```python
from build123d import *

# Parameters (mm, degrees)
BOSS_EXTRUDE2_DEPTH            = 30
BOSS_EXTRUDE2_DEPTH_BACK       = 30
EXTRUDE_THIN2_START            = -25
EXTRUDE_THIN2_DEPTH            = 50
SKETCH2_W                      = 60
SKETCH2_H                      = 5
BOSS_EXTRUDE3_DEPTH            = 100
BOSS_EXTRUDE4_DEPTH            = 30
BOSS_EXTRUDE4_DEPTH_BACK       = 30
CUT_EXTRUDE2_REACH             = 143.361
SKETCH4_W                      = 60
SKETCH4_H                      = 5
CUT_EXTRUDE2_DIRECTION_2_REACH = 143.361
BOSS_EXTRUDE5_DEPTH            = 30
BOSS_EXTRUDE5_DEPTH_BACK       = 30
DRONE_ARM_FIT_CUT_DEPTH        = 50
CUT_EXTRUDE3_START             = -60
SKETCH8_W                      = 5
SKETCH8_H                      = 5
CUT_EXTRUDE3_DEPTH             = 60
SKETCH10_R                     = 13.15
CUT_EXTRUDE5_DEPTH             = 60


# Read off the part's stored shape, not the designer's step: Extrude-Thin2
with BuildPart() as part:
    # Sketch1 → Boss-Extrude2 (new, two sides: drawn at the far end of the back side and taken through both)
    with BuildSketch(Plane.XY.offset(-BOSS_EXTRUDE2_DEPTH_BACK)):
        Polygon((-13.01396445, -23.830717844), (13.01396445, -23.830717844), (55, -0.089432632), (55, 13.432214294), (-55, 13.432214294), (-55, -0.089432632), align=None)
    extrude(amount=BOSS_EXTRUDE2_DEPTH + BOSS_EXTRUDE2_DEPTH_BACK)

    # Extrude-Thin2 outline → Extrude-Thin2 (add)
    with BuildSketch(Plane.XY.offset(EXTRUDE_THIN2_START)):
        Polygon((50, 13.432214294), (55, 13.432214294), (55, 68.432214294), (-55, 68.432214294), (-55, 13.432214294), (-50, 13.432214294), (-50, 63.432214294), (50, 63.432214294), align=None)
    extrude(amount=EXTRUDE_THIN2_DEPTH)

    # Sketch2 → Boss-Extrude3 (add)
    with BuildSketch(Plane.ZY.offset(-50)):
        with Locations((0, 37.694873029)):
            Rectangle(SKETCH2_W, SKETCH2_H)
    extrude(amount=BOSS_EXTRUDE3_DEPTH)

    # Sketch1<6> → Boss-Extrude4 (add, two sides: drawn at the far end of the back side and taken through both)
    with BuildSketch(Plane.XY.offset(-BOSS_EXTRUDE4_DEPTH_BACK)):
        Polygon((-55, -0.089432632), (-55, 13.432214294), (-70, 13.432214294), (-70, -8.839581066), (-16.961214453, -38.830717844), (16.961214453, -38.830717844), (70, -8.839581066), (70, 13.432214294), (55, 13.432214294), (55, -0.089432632), (13.01396445, -23.830717844), (-13.01396445, -23.830717844), align=None)
    extrude(amount=BOSS_EXTRUDE4_DEPTH + BOSS_EXTRUDE4_DEPTH_BACK)

    # Cut-Extrude2: up to this face of the body (flat: up to its plane)
    cut_extrude2_end = Plane(part.part.faces().sort_by_distance((-55, 40.932214294, 0))[0])
    # Sketch4 → Cut-Extrude2 (cut, up to the picked face)
    with BuildSketch(Plane(origin=(-50, 0, 0), x_dir=(0, 0, -1), z_dir=(1, 0, 0)), mode=Mode.PRIVATE) as cut_extrude2_sk1:
        with Locations((0, 65.932214294)):
            Rectangle(SKETCH4_W, SKETCH4_H)
    cut_extrude2_tool1 = split(extrude(cut_extrude2_sk1.sketch, amount=-CUT_EXTRUDE2_REACH, mode=Mode.PRIVATE), bisect_by=cut_extrude2_end, keep=Keep.BOTH, mode=Mode.PRIVATE)
    add(cut_extrude2_tool1.solids().sort_by(Axis((-50, 65.932214, 0), (-1, 0, 0)))[0], mode=Mode.SUBTRACT)

    # Cut-Extrude2 direction 2: up to this face of the body (flat: up to its plane)
    cut_extrude2_direction_2_end = Plane(part.part.faces().sort_by_distance((55, 40.932214294, 0))[0])
    # Sketch4 → Cut-Extrude2 direction 2 (cut, up to the picked face)
    with BuildSketch(Plane(origin=(-50, 0, 0), x_dir=(0, 0, -1), z_dir=(1, 0, 0)), mode=Mode.PRIVATE) as cut_extrude2_direction_2_sk1:
        with Locations((0, 65.932214294)):
            Rectangle(SKETCH4_W, SKETCH4_H)
    cut_extrude2_direction_2_tool1 = split(extrude(cut_extrude2_direction_2_sk1.sketch, amount=CUT_EXTRUDE2_DIRECTION_2_REACH, mode=Mode.PRIVATE), bisect_by=cut_extrude2_direction_2_end, keep=Keep.BOTH, mode=Mode.PRIVATE)
    add(cut_extrude2_direction_2_tool1.solids().sort_by(Axis((-50, 65.932214, 0), (1, 0, 0)))[0], mode=Mode.SUBTRACT)

    # Sketch1<7> → Boss-Extrude5 (add, two sides: drawn at the far end of the back side and taken through both)
    with BuildSketch(Plane.XY.offset(-BOSS_EXTRUDE5_DEPTH_BACK)):
        Polygon((-70, 13.432214294), (-55, 13.432214294), (-50, 13.432214294), (-50, 38.432214294), (-50, 63.432214294), (-70, 63.432214294), (-70, 38.432214294), align=None)
        Polygon((50, 38.432214294), (50, 13.432214294), (55, 13.432214294), (70, 13.432214294), (70, 38.432214294), (70, 63.432214294), (50, 63.432214294), align=None)
    extrude(amount=BOSS_EXTRUDE5_DEPTH + BOSS_EXTRUDE5_DEPTH_BACK)

    # Sketch7 → Drone Arm fit cut (cut)
    with BuildSketch(Plane(origin=(0, 63.432214294, 0), x_dir=(1, 0, 0), z_dir=(0, 1, 0))):
        Polygon((-70, -12.7), (-70, 12.7), (-65, 12.7), (-65, 7.7), (-60, 7.7), (-60, 12.7), (-60, 17.5), (-55, 17.5), (-55, -17.5), (-60, -17.5), (-60, -12.7), (-60, -7.7), (-65, -7.7), (-65, -12.7), align=None)
    drone_arm_fit_cut = extrude(amount=-DRONE_ARM_FIT_CUT_DEPTH, mode=Mode.SUBTRACT)

    # Mirror Drone arm fit cut: Drone Arm fit cut across plane
    add(drone_arm_fit_cut.mirror(Plane(origin=(0, 0, 0), x_dir=(0, 0, 1), z_dir=(1, 0, 0))), mode=Mode.SUBTRACT)

    # Sketch8 → Cut-Extrude3 (cut)
    with BuildSketch(Plane.XY.offset(30).offset(CUT_EXTRUDE3_START)):
        with Locations((-60, 50.932214294)):
            Rectangle(SKETCH8_W, SKETCH8_H)
        with Locations((-60, 30.932214294)):
            Rectangle(SKETCH8_W, SKETCH8_H)
    cut_extrude3 = extrude(amount=CUT_EXTRUDE3_DEPTH, mode=Mode.SUBTRACT)

    # Mirror1: Cut-Extrude3 across plane
    add(cut_extrude3.mirror(Plane(origin=(0, 0, 0), x_dir=(0, 0, 1), z_dir=(1, 0, 0))), mode=Mode.SUBTRACT)

    # Sketch10 → Cut-Extrude5 (cut)
    with BuildSketch(Plane.XY.offset(30)):
        with Locations((0, -7.922241987)):
            Circle(SKETCH10_R)
    extrude(amount=-CUT_EXTRUDE5_DEPTH, mode=Mode.SUBTRACT)


solid = part.part
```
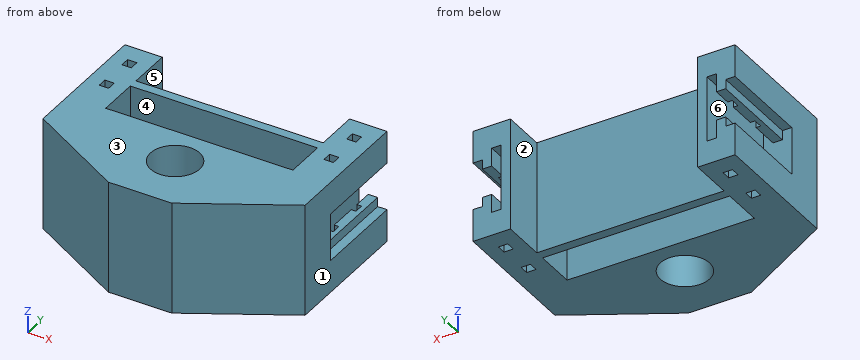
Verification items for the finished model (mm, model axes). Face numbers are marked on the shaded views. A direction names the side the tool comes from. Give positions to 0.01 mm unless a question says otherwise; leave off trailing zeros. Order: outer loops, then holes, each group sorted by start corner. A loop starts at its lowest first (then second) coordinate and runs counter-clockwise, first axis right, second up. Notation, with made-up numbers: (-34, -32.75) -> (-14, -32.75) arc R17 ccw to (-14, -27.75) -> close; hole circle Ø3 at (17.25, -10.75). An arc over 180 degrees is marked (long way). Use a Markdown table: item, result.
1) Section check C-C, the plane z = -21.5. Give the number of separate pieces and of enclosed holes in the cut face, then the cut area to 3 significant figures.
Results:
| item | result |
|---|---|
| separate pieces | 1 |
| enclosed holes | 6 |
| area | 7,580 mm² |
2) Section check B-B, the plane y = 2. Record the boundary of the cut face in (x, z).
Results:
| item | result |
|---|---|
| outline | (-70, -30) -> (-8.63, -30) -> (-8.63, 30) -> (-70, 30) -> close; (8.63, -30) -> (70, -30) -> (70, 30) -> (8.63, 30) -> close |
3) Depth check by flat-ended pin: pin 1 Ø1.5 at (x, z) = (23, -24) entering from -Y; pin 2 Ø2.5 at (y, z) = (36.5, -9.5) entering from +X; pin 3 Ø12 at (x, z) = (-17.5, 12) entering from +Y; pin 4 Ø23.5 at (x, y) = (0, -7.92) entering from -Z. Enter the tip coordinate at first touch or a pass-through.
Results:
| item | result |
|---|---|
| pin 1 | y = -35.84 |
| pin 2 | x = 65 |
| pin 3 | y = 40.19 |
| pin 4 | through |
4) Tool access check on the marked faces 4, 5 and 6. Record the directions out of +Z, -Z, +X, -X, +Y, -Y that give a thin tool (end or side, any length) a straight path to the whole face; none if there is none.
Results:
| item | result |
|---|---|
| face 4 | +Z, -Z |
| face 5 | +Z, -Z, +Y |
| face 6 | +Y |
5) Section check A-A, the plane x = 0. Record the boundary of the cut face in (y, z), then the cut area to 3 significant figures.
Results:
| item | result |
|---|---|
| outline | (-38.83, -30) -> (-21.07, -30) -> (-21.07, 30) -> (-38.83, 30) -> close; (5.23, -30) -> (13.43, -30) -> (13.43, 30) -> (5.23, 30) -> close; (35.19, -30) -> (40.19, -30) -> (40.19, 30) -> (35.19, 30) -> close |
| area | 1,860 mm² |
6) Mould release check, pull along X, two halves, no side actions. Record for the marked faces 1, 2 and 3: pulls with the +X half, pulls with the -X half, needs draft (parallel to the pull), parting line crosses it, or undercut.
Results:
| item | result |
|---|---|
| face 1 | pulls with the +X half |
| face 2 | undercut |
| face 3 | needs draft |
7) Section check D-D, the plane x = 48. Record the boundary of the cut face in (y, z).
Results:
| item | result |
|---|---|
| outline | (-21.28, -30) -> (13.43, -30) -> (13.43, 30) -> (-21.28, 30) -> close; (35.19, -30) -> (40.19, -30) -> (40.19, 30) -> (35.19, 30) -> close |
8) Material ranges on probe 1 along X at (y, z) = (45, 8); probe 2 along Y at (x, z) = (0, -14); probe 3 along X at (y, z) = (41, -23), recorded low to high.
Results:
| item | result |
|---|---|
| probe 1 | -65 to -60, -55 to -50, 50 to 55, 60 to 65 |
| probe 2 | -38.83 to -21.07, 5.23 to 13.43, 35.19 to 40.19 |
| probe 3 | -70 to -50, 50 to 70 |
